Build history of the part. All positions in model axes, mm. Face numbers are marked on the shaded views. Coordinates: 2 decimals unless noted, no trailing zeros. Order: outer loops, then holes, each group sorted by start corner. A loop starts at its lowest first (then second) coordinate and runs counter-clockwise, first axis right, second up. Notation, with made-up numbers: (77.25, 66.25) -> (115.25, 66.25) arc R23 ccw to (115.25, 97.25) -> close; hole circle Ø3 at (83.25, 44). An arc over 180 degrees is marked (long way). Write each question's results on one line, items separated by ' | '.
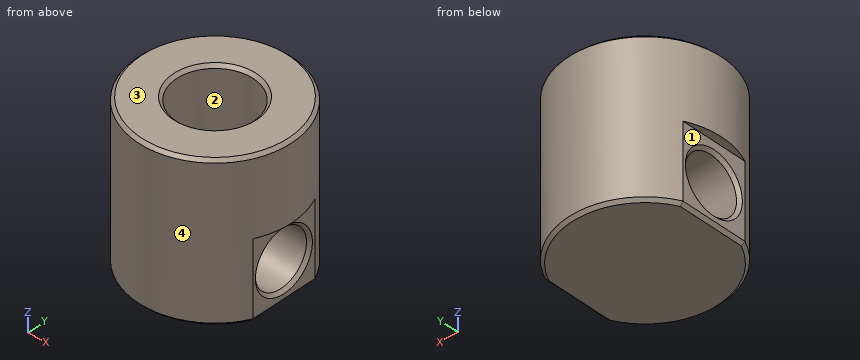
from build123d import *

# Parameters (mm, degrees)
F0_R     = 25
F1_DEPTH = 50
F2_W     = 23.745389397
F2_H     = 47.3247256844
F2_W_2   = 14.1143929356
F3_DEPTH = 25
F5_D     = 18
F6_R     = 12.5
F7_DEPTH = 25
F8_SIZE  = 1


with BuildPart() as f1:
    # F0 (on Top) → F1 (new body)
    with BuildSketch(Plane.XY):
        Circle(F0_R)
    extrude(amount=F1_DEPTH)

    # F2 (on Top) → F3 (cut)
    with BuildSketch(Plane.XY):
        with Locations((34.3726946985, 1.0396027938)):
            Rectangle(F2_W, F2_H)
        with Locations((-29.5571964678, 1.0396027938)):
            Rectangle(F2_W_2, F2_H)
    extrude(amount=F3_DEPTH, mode=Mode.SUBTRACT)

    # F5 (through all)
    with Locations(Plane.YZ.offset(22.5)):
        with Locations((0, 12.5)):
            Hole(F5_D / 2)

    # F6 (on face) → F7 (cut)
    with BuildSketch(Plane.XY.offset(50)):
        Circle(F6_R)
    extrude(amount=-F7_DEPTH, mode=Mode.SUBTRACT)

    # F8
    f8_edges = [f1.edges().sort_by_distance(p)[0] for p in [
        (-25, 0, 50),
        (0, 25, 0),
        (0, -25, 0),
        (22.5, 0, 0),
        (-22.5, 0, 0),
        (-12.5, 0, 50),
        (22.5, -9, 12.5),
        (-22.5, -9, 12.5),
    ]]
    chamfer(f8_edges, length=F8_SIZE)


solid = f1.part
Item 1: Slice it at D-D, the plane z = 39. List the corners of the cut face in (x, y).
Answer:
outline: circle Ø50 at (0, 0); hole circle Ø25 at (0, 0)
Item 2: Drill centre lines: line 1 (Y direction, x = 0, z = 43); line 2 (X direction, y = 11, z = 29); line 3 (Y direction, x = -19, z = 16). Where is each one in solid material? Low to high. Write a range as from..to.
Answer:
line 1: y = -25..-12.5, 12.5..25 | line 2: x = -22.45..-5.94, 5.94..22.45 | line 3: y = -16.25..-8.29, 8.29..16.25
Item 3: Slice it at A-A, the plane z = 12.5. List the corners of the cut face in (x, y).
Answer:
outline: (-22.5, -10.9) arc R25 ccw to (22.5, -10.9) -> (22.5, -10) -> (21.5, -9) -> (-21.5, -9) -> (-22.5, -10) -> close; (-22.5, 10) -> (-21.5, 9) -> (21.5, 9) -> (22.5, 10) -> (22.5, 10.9) arc R25 ccw to (-22.5, 10.9) -> close
Item 4: Slice it at C-C, the plane x = 0. List the corners of the cut face in (y, z), and give its area (3 significant figures).
Answer:
outline: (-25, 1) -> (-24, 0) -> (24, 0) -> (25, 1) -> (25, 49) -> (24, 50) -> (13.5, 50) -> (12.5, 49) -> (12.5, 25) -> (-12.5, 25) -> (-12.5, 49) -> (-13.5, 50) -> (-24, 50) -> (-25, 49) -> close; hole circle Ø18 at (0, 12.5) | area: 1,620 mm^2
Item 5: Pin check, flat tips, straight feed: pin 1 (5 mm diameter, centred on y = -18, z = 11.5, fed in from +X); pin 2 (4 mm diameter, centred on x = 1.5, z = 15, fed in from +Y); pin 3 (1 mm diameter, centred on x = 4, z = 22.5, fed in from +Y); pin 4 (11 mm diameter, centred on y = 0, z = 12.5, fed in from -X). Stop position of each tip, or through.
Answer:
pin 1: stops at x = 19.62 | pin 2: stops at y = 25 | pin 3: stops at y = 24.75 | pin 4: passes through
Item 6: Pull direction X, two halves, no side cores. Call the marked faces 1, 2, 3 and 4: released by +X, released by -X, zero draft, split by the parting line, or undercut.
Answer:
face 1: released by -X | face 2: undercut | face 3: zero draft | face 4: split by the parting line
Item 7: Slice it at B-B, the plane y = 0. List the corners of the cut face in (x, z), and give its area (3 significant figures).
Answer:
outline: (-25, 25) -> (-22.5, 25) -> (-22.5, 22.5) -> (-21.5, 21.5) -> (21.5, 21.5) -> (22.5, 22.5) -> (22.5, 25) -> (25, 25) -> (25, 49) -> (24, 50) -> (13.5, 50) -> (12.5, 49) -> (12.5, 25) -> (-12.5, 25) -> (-12.5, 49) -> (-13.5, 50) -> (-24, 50) -> (-25, 49) -> close; (-22.5, 1) -> (-21.5, 0) -> (21.5, 0) -> (22.5, 1) -> (22.5, 2.5) -> (21.5, 3.5) -> (-21.5, 3.5) -> (-22.5, 2.5) -> close | area: 935 mm^2
